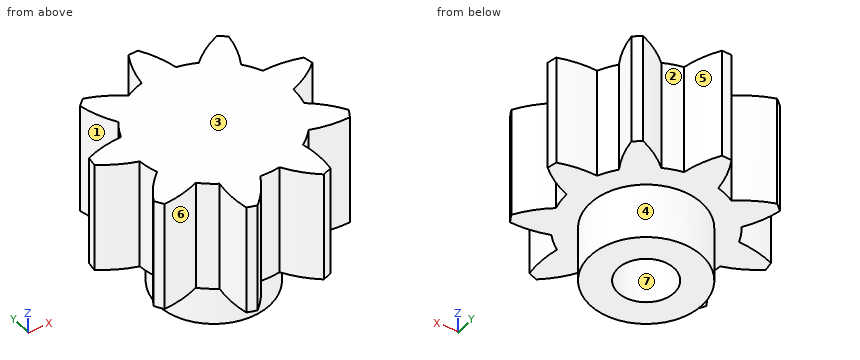
from build123d import *

# Parameters (mm, degrees)
ESQUISSE1_R                  = 10
BOSS_EXTRU_1_DEPTH           = 10
ESQUISSE2_R                  = 5
BOSS_EXTRU_2_DEPTH           = 5
ESQUISSE3_R                  = 2.5
ENL_V_MAT_EXTRU_2_DEPTH      = 5
ENL_V_START                  = -10
ENL_V_MAT_EXTRU_4_DEPTH      = 10
R_P_TITION_CIRCULAIRE2_COUNT = 9


with BuildPart() as part:
    # Esquisse1 → Boss.-Extru.1 (new body)
    with BuildSketch(Plane.XY):
        Circle(ESQUISSE1_R)
    extrude(amount=BOSS_EXTRU_1_DEPTH)

    # Esquisse2 → Boss.-Extru.2 (add)
    with BuildSketch(Plane(origin=(0, 0, 0), x_dir=(-1, 0, 0), z_dir=(0, 0, -1))):
        Circle(ESQUISSE2_R)
    extrude(amount=BOSS_EXTRU_2_DEPTH)

    # Esquisse3 → Enlèv. mat.-Extru.2 (cut)
    with BuildSketch(Plane(origin=(0, 0, -5), x_dir=(-1, 0, 0), z_dir=(0, 0, -1))):
        Circle(ESQUISSE3_R)
    extrude(amount=-ENL_V_MAT_EXTRU_2_DEPTH, mode=Mode.SUBTRACT)

    # Esquisse5 → Enlèv. mat.-Extru.4 (cut)
    with BuildSketch(Plane.XY.offset(10).offset(ENL_V_START)):
        with BuildLine():
            ThreePointArc((0, 10), (0.771400633, 8.500970859), (1.256296491, 6.886342943))
            ThreePointArc((1.256296491, 6.886342943), (2.104940597, 6.676018655), (2.920746205, 6.361543964))
            ThreePointArc((2.920746205, 6.361543964), (4.244062165, 7.406044884), (5.735764364, 8.191520443))
            ThreePointArc((5.735764364, 8.191520443), (3.007057995, 9.537169507), (0, 10))
        make_face()
    enl_v_mat_extru_4 = extrude(amount=ENL_V_MAT_EXTRU_4_DEPTH, mode=Mode.SUBTRACT)

    # Répétition circulaire2: Enlèv. mat.-Extru.4 ×9 about axis
    r_p_tition_circulaire2_axis = Axis((0, 0, 0), (0, 0, 1))
    for i in range(1, R_P_TITION_CIRCULAIRE2_COUNT):
        add(enl_v_mat_extru_4.rotate(r_p_tition_circulaire2_axis, i * 360 / R_P_TITION_CIRCULAIRE2_COUNT), mode=Mode.SUBTRACT)


solid = part.part
Design review of the part built by this model. Coordinates are the model's own, in mm. Face numbers are marked on the shaded views. A direction names the side the tool comes from. Give positions to 0.01 mm unless a question says otherwise; leave off trailing zeros. Loops run counter-clockwise (first coordinate to the right, second up) from the corner with the lowest first, then second, coordinate; pieces in that order, holes last. Notation, with made-up numbers: M 42.25,63 L 96.25,63 A16 cw 96.25,92 Z; hole C 1.5,58 d8. An arc over 180 degrees is marked long. Answer as a JSON object with one key per item and string values.
Item 1: We need section A-A (z = -3.25). State the section outline as (x, y) points.
Output values:
{"outline": "C 0,0 d10; hole C 0,0 d5"}
Item 2: We need section C-C (y = -8). State the section outline as (x, z) points, and give its area (3 significant figures).
Output values:
{"outline": "M -3.62,0 L -1.16,0 L -1.16,10 L -3.62,10 Z; M 1.96,0 L 4.3,0 L 4.3,10 L 1.96,10 Z", "area": "48.0 mm2"}
Item 3: For P1, Ø1.5, axis at x = 0.5, y = -0.5, coming from the -Z side; P2, Ø8, axis at y = -7.5, z = 1.5, coming from the +X side; P3, Ø1.5, axis at x = -7, z = -1, coming from the -Y side; P4, Ø1.5, axis at y = 0, z = 4.5, coming from the +X side, all flat-tipped, find the tip position at first contact; note any pin that passes through.
Output values:
{"P1": "stops at z = 0", "P2": "stops at x = 9.06", "P3": "passes through", "P4": "stops at x = 8.56"}
Item 4: We need section D-D (y = 5.5). State the section outline as (x, z) points.
Output values:
{"outline": "M -6.57,0 L 5.87,0 L 5.87,10 L -6.57,10 Z"}
Item 5: Machinability: for the marked faces 5, 6 and 7, which of the approach directions +Z, -Z, +X, -X, +Y, -Y give a long, thin tool a straight path to every point of the face, cutting with its end or side? Answer none if there is none.
Output values:
{"face 5": "+Z, -Z, +Y", "face 6": "+Z, -Z, -Y", "face 7": "-Z"}
Item 6: Mouldability with a two-part tool opening along X and no side actions: class the marked faces 1, 2, 3 and 4 as pulls with the +X half, pulls with the -X half, needs draft (parallel to the pull), parting line crosses it, or undercut.
Output values:
{"face 1": "pulls with the -X half", "face 2": "undercut", "face 3": "needs draft", "face 4": "parting line crosses it"}
Item 7: Wall thickness on line 1 along Y through (x, z) = (0, -2.15); line 2 along Z through (x, y) = (6.75, -4.5); line 3 along X through (y, z) = (-2.25, -2): over which ranges is each line inside the solid? List them lowest first.
Output values:
{"line 1": "y = -5 to -2.5, 2.5 to 5", "line 2": "z = 0 to 10", "line 3": "x = -4.47 to -1.09, 1.09 to 4.47"}
Item 8: We need section B-B (x = -7.75). State the section outline as (y, z) points.
Output values:
{"outline": "M -5.71,0 L -3.59,0 L -3.59,10 L -5.71,10 Z; M -0.38,0 L 2.33,0 L 2.33,10 L -0.38,10 Z"}
